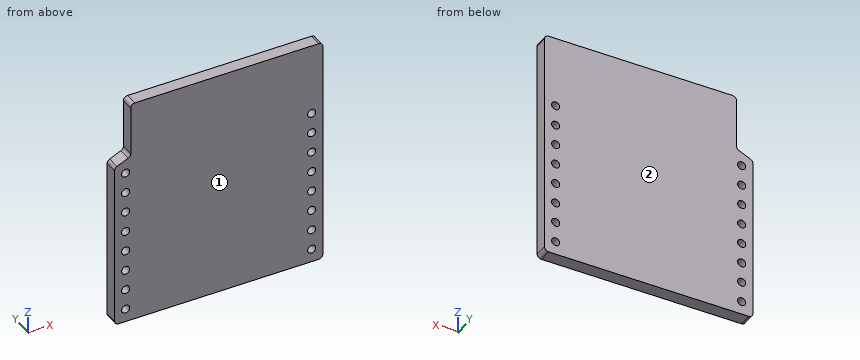
from build123d import *

# Parameters (mm, degrees)
SKETCH2_R           = 0.5
BOSS_EXTRUDE1_DEPTH = 1.6
FILLET1_R           = 0.5


with BuildPart() as part:
    # Sketch2 → Boss-Extrude1 (new body)
    with BuildSketch(Plane(origin=(0, 0, 0), x_dir=(1, 0, 0), z_dir=(0, 1, 0))):
        Polygon((-12.8, 7.690457371), (-12.8, 28.2), (12.8, 28.2), (12.8, 0), (-10.8, 0), (-10.8, 6.8), align=None)
        with Locations((-11.43, 26.58)):
            Circle(SKETCH2_R, mode=Mode.SUBTRACT)
        with Locations((11.43, 26.58)):
            Circle(SKETCH2_R, mode=Mode.SUBTRACT)
        with Locations((-11.43, 24.04)):
            Circle(SKETCH2_R, mode=Mode.SUBTRACT)
        with Locations((11.43, 24.04)):
            Circle(SKETCH2_R, mode=Mode.SUBTRACT)
        with Locations((-11.43, 21.5)):
            Circle(SKETCH2_R, mode=Mode.SUBTRACT)
        with Locations((11.43, 21.5)):
            Circle(SKETCH2_R, mode=Mode.SUBTRACT)
        with Locations((-11.43, 18.96)):
            Circle(SKETCH2_R, mode=Mode.SUBTRACT)
        with Locations((11.43, 18.96)):
            Circle(SKETCH2_R, mode=Mode.SUBTRACT)
        with Locations((-11.43, 16.42)):
            Circle(SKETCH2_R, mode=Mode.SUBTRACT)
        with Locations((11.43, 16.42)):
            Circle(SKETCH2_R, mode=Mode.SUBTRACT)
        with Locations((-11.43, 13.88)):
            Circle(SKETCH2_R, mode=Mode.SUBTRACT)
        with Locations((11.43, 13.88)):
            Circle(SKETCH2_R, mode=Mode.SUBTRACT)
        with Locations((-11.43, 11.34)):
            Circle(SKETCH2_R, mode=Mode.SUBTRACT)
        with Locations((11.43, 11.34)):
            Circle(SKETCH2_R, mode=Mode.SUBTRACT)
        with Locations((-11.43, 8.8)):
            Circle(SKETCH2_R, mode=Mode.SUBTRACT)
        with Locations((11.43, 8.8)):
            Circle(SKETCH2_R, mode=Mode.SUBTRACT)
    extrude(amount=BOSS_EXTRUDE1_DEPTH)

    # Fillet1
    fillet1_edges = [part.edges().sort_by_distance(p)[0] for p in [
        (12.8, 0.8, 0),
        (-10.8, 0.8, 0),
        (-10.8, 0.8, -6.8),
        (-12.8, 0.8, -7.690457371),
        (-12.8, 0.8, -28.2),
        (12.8, 0.8, -28.2),
    ]]
    fillet(fillet1_edges, radius=FILLET1_R)


solid = part.part
Source: CAD feature listing. Evaluate the final solid. Frame: model axes, mm. Face numbers are marked on the shaded views. Round coordinates to 2 decimals unless told otherwise and drop trailing zeros. Write each loop counter-clockwise with the first axis right and the second up, starting at its lowest first coordinate (ties: lowest second). Pieces come first, ordered by that corner, then holes. Notation, with made-up numbers: (15.5, 57) - (57.5, 57) arc R33 cw to (57.5, 92) - close; hole circle Ø2 at (-7, 4). An arc over 180 degrees is marked (long way). Use CSV: the item, a comma, the result in double quotes. Start each with the question number.
(1) Cut plane A-A, the plane y = 1. Give the number of separate pieces and of enclosed holes in the cut face, and give its area (3 significant figures).
(2) Cut plane B-B, the plane z = -18.96. Return loops of the section in (x, y), and give its area (3 significant figures).
(3) Material intervals for probe 1 along X at (y, z) = (0.4, -18.96); probe 2 along X at (y, z) = (1.1, -8.5); probe 3 along X at (y, z) = (0.9, -1), sorted ascending. Write a range as [from, to].
(4) First-contact query: pin 1 Ø6 at (x, z) = (-5.5, -9) entering from -Y. Flat tip, straight axial feed; report the tip coordinate or a pass-through.
(5) Mould query, pull axis Y, two halves, no side actions, for the marked faces 1 and 2. Classes: pulls with the +Y half, pulls with the -Y half, needs draft (parallel to the pull), parting line crosses it, or undercut.
Geometry says:
1,separate pieces,"1"
1,enclosed holes,"16"
1,area,"695 mm²"
2,outline,"(-12.8, 0) - (-11.93, 0) - (-11.93, 1.6) - (-12.8, 1.6) - close; (-10.93, 0) - (10.93, 0) - (10.93, 1.6) - (-10.93, 1.6) - close; (11.93, 0) - (12.8, 0) - (12.8, 1.6) - (11.93, 1.6) - close"
2,area,"37.8 mm²"
3,probe 1,"[-12.8, -11.93], [-10.93, 10.93], [11.93, 12.8]"
3,probe 2,"[-12.8, -11.83], [-11.03, 11.03], [11.83, 12.8]"
3,probe 3,"[-10.8, 12.8]"
4,pin 1,"y = 0"
5,face 1,"pulls with the -Y half"
5,face 2,"pulls with the +Y half"
